For this review, take the finished solid that the model builds, in its own axes (mm). Give positions to 0.01 mm unless a question says otherwise; leave off trailing zeros. Order: outer loops, then holes, each group sorted by start corner. A loop starts at its lowest first (then second) coordinate and runs counter-clockwise, first axis right, second up. Notation, with made-up numbers: (-24, 41.5) - (29, 41.5) arc R34 cw to (29, 79.5) - close; hole circle Ø4 at (10, 71.25). An arc over 180 degrees is marked (long way). One line per item, written item: value.
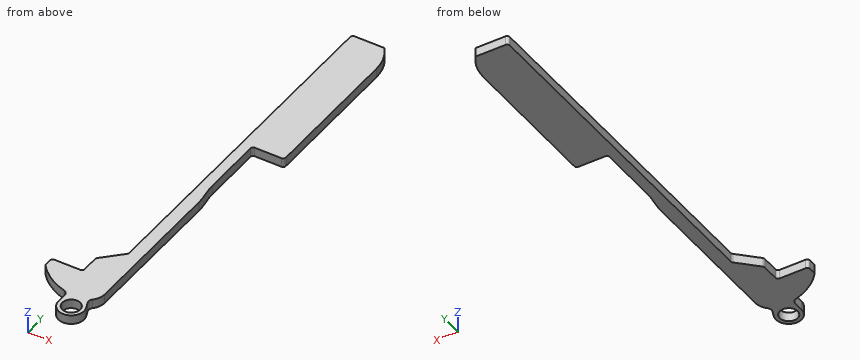
```python
from build123d import *

# Parameters (mm, degrees)
BOSS_EXTRUDE1_DEPTH = 1.8
FILLET1_R           = 0.5
SKETCH5_R           = 2.5
SKETCH5_R_2         = 1.75
BOSS_EXTRUDE2_DEPTH = 1.8
FILLET2_R           = 1


with BuildPart() as part:
    # Sketch1 → Boss-Extrude1 (new body)
    with BuildSketch(Plane.XY):
        with BuildLine():
            Line((0, 4.5), (0, 6.5))
            Line((0, 6.5), (6.1, 6.5))
            Line((6.1, 6.5), (6.1, 10.5))
            Line((6.1, 10.5), (10, 14.4))
            Line((10, 14.4), (10, 83.5))
            Line((10, 83.5), (16.4, 83.5))
            ThreePointArc((16.4, 83.5), (17.745328581, 80.945017946), (18.212299295, 78.095495067))
            Line((18.212299295, 78.095495067), (18.25, 49.5))
            Line((18.25, 49.5), (12, 49.5))
            Line((12, 49.5), (12, 37.18))
            add(Edge.make_bspline(
                [(12, 37.18), (12, 35.554764974), (12.5, 33.972282338), (12.5, 32.33)],
                knots=[0, 0, 0, 0, 1, 1, 1, 1], degree=3))
            Line((12.5, 32.33), (12.5, 3.07))
            ThreePointArc((12.5, 3.07), (11.600817818, 0.899182182), (9.43, 0))
            ThreePointArc((9.43, 0), (4.205660329, 1.182650422), (0, 4.5))
        make_face()
    extrude(amount=BOSS_EXTRUDE1_DEPTH)

    # Fillet1
    fillet1_edges = [part.edges().sort_by_distance(p)[0] for p in [
        (0, 6.5, 0.9),
        (6.1, 6.5, 0.9),
        (6.1, 10.5, 0.9),
        (10, 14.4, 0.9),
        (10, 83.5, 0.9),
        (18.25, 49.5, 0.9),
        (12, 49.5, 0.9),
    ]]
    fillet(fillet1_edges, radius=FILLET1_R)

    # Sketch5 → Boss-Extrude2 (add)
    # profile 1 of 3: a face of its own
    with BuildSketch(Plane(origin=(0, 0, 0), x_dir=(-1, 0, 0), z_dir=(0, 0, -1))):
        with Locations((-9.5, -2.499832541)):
            Circle(SKETCH5_R)
        with Locations((-9.5, -2.499832541)):
            Circle(SKETCH5_R_2, mode=Mode.SUBTRACT)
    # profile 2 of 3: a face of its own
    with BuildSketch(Plane(origin=(0, 0, 0), x_dir=(-1, 0, 0), z_dir=(0, 0, -1))):
        with BuildLine():
            ThreePointArc((-11.824045318, -1.578521867), (-9.031018815, -0.044215175), (-7, -2.499832541))
            Line((-7, -2.499832541), (-7, 0.245881701))
            ThreePointArc((-7, 0.245881701), (-8.2087959, 0.061626967), (-9.43, 0))
            ThreePointArc((-9.43, 0), (-10.256451345, 0.113333266), (-11.021883517, 0.444965358))
            Line((-11.021883517, 0.444965358), (-11.824045318, -1.578521867))
        make_face()
    # profile 3 of 3: a face of its own
    with BuildSketch(Plane(origin=(0, 0, 0), x_dir=(-1, 0, 0), z_dir=(0, 0, -1))):
        with BuildLine():
            ThreePointArc((-9.43, 0), (-8.2087959, 0.061626967), (-7, 0.245881701))
            Line((-7, 0.245881701), (-7, 0.500167459))
            Line((-7, 0.500167459), (-11, 0.500167459))
            Line((-11, 0.500167459), (-11.021883517, 0.444965358))
            ThreePointArc((-11.021883517, 0.444965358), (-10.256451345, 0.113333266), (-9.43, 0))
        make_face()
    extrude(amount=-BOSS_EXTRUDE2_DEPTH)

    # Fillet2
    fillet2_edges = [part.edges().sort_by_distance(p)[0] for p in [
        (7, 0.245881701, 0.9),
        (11.021883517, 0.444965358, 0.9),
    ]]
    fillet(fillet2_edges, radius=FILLET2_R)


solid = part.part
```
(1) Take a section at A-A (y = 8). Write out the cut boundary in (x, z), then the cut area to 3 significant figures.
Answers below:
outline: (6.1, 0) - (12.5, 0) - (12.5, 1.8) - (6.1, 1.8) - close
area: 11.5 mm^2
(2) Wall thickness on line 1 (X direction, y = 50.5, z = 0.25); line 2 (X direction, y = 47, z = 0.6); line 3 (Y direction, x = 11, z = 0.7): over which ranges is each line inside the solid? List them lowest first. Write a range as from..to.
Answers below:
line 1: x = 10..18.25
line 2: x = 10..12
line 3: y = -4.5..-3.4, -1.6..83.5
(3) For P1, Ø0.9, axis at y = 44, z = 1, coming from the +X side; P2, Ø1, axis at y = 16.5, z = 1, coming from the -X side, all flat-tipped, find the tip position at first contact; note any pin that passes through.
Answers below:
P1: stops at x = 12
P2: stops at x = 10
(4) Take a section at B-B (x = 14.25). Write out the cut boundary in (y, z).
Answers below:
outline: (49.5, 0) - (83.5, 0) - (83.5, 1.8) - (49.5, 1.8) - close
